Read the model definition and answer for the solid it produces. Units are mm, in the model's axes. Face numbers are marked on the shaded views. A direction names the side the tool comes from. Coordinates: 2 decimals unless noted, no trailing zeros. Loops run counter-clockwise (first coordinate to the right, second up) from the corner with the lowest first, then second, coordinate; pieces in that order, holes last.
from build123d import *

# Parameters (mm, degrees)
F0_W     = 127
F0_H     = 38.1
F1_DEPTH = 25.4
F4_DEPTH = 38.1
F5_DEPTH = 38.1
F3_R     = 6.35
F6_DEPTH = 25.4


with BuildPart() as f1:
    # F0 (on Top) → F1 (new body)
    with BuildSketch(Plane.XY):
        with Locations((3.767781, -13.309208)):
            Rectangle(F0_W, F0_H)
    extrude(amount=F1_DEPTH)

    # F2 (on face) → F4 (join)
    with BuildSketch(Plane.XZ.offset(32.359208)):
        with BuildLine():
            Line((-25.331575, 25.4), (-8.932219, 25.4))
            ThreePointArc((-8.932219, 25.4), (3.767781, 38.1), (16.467781, 25.4))
            Line((16.467781, 25.4), (32.867137, 25.4))
            ThreePointArc((32.867137, 25.4), (25.91106, 27.474418), (21.227394, 33.02))
            ThreePointArc((21.227394, 33.02), (3.767781, 44.45), (-13.691832, 33.02))
            ThreePointArc((-13.691832, 33.02), (-18.375498, 27.474418), (-25.331575, 25.4))
        make_face()
    extrude(amount=-F4_DEPTH)

    # F2 (on face) → F5 (cut)
    with BuildSketch(Plane.XZ.offset(32.359208)):
        with BuildLine():
            ThreePointArc((-8.932219, 25.4), (-5.212475, 16.419744), (3.767781, 12.7))
            Line((3.767781, 12.7), (3.767781, 25.4))
            Line((3.767781, 25.4), (-8.932219, 25.4))
        make_face()
        with BuildLine():
            Line((3.767781, 25.4), (3.767781, 12.7))
            ThreePointArc((3.767781, 12.7), (12.748037, 16.419744), (16.467781, 25.4))
            Line((16.467781, 25.4), (3.767781, 25.4))
        make_face()
    extrude(amount=-F5_DEPTH, mode=Mode.SUBTRACT)

    # F3 (on face) → F6 (cut)
    with BuildSketch(Plane.XY.offset(25.4)):
        with Locations((-40.682219, -13.309208)):
            Circle(F3_R)
        with Locations((48.217781, -13.309208)):
            Circle(F3_R)
    extrude(amount=-F6_DEPTH, mode=Mode.SUBTRACT)


solid = f1.part
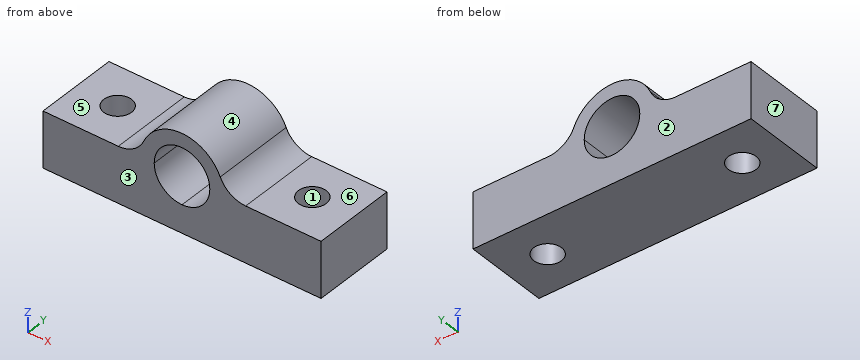
Q1. A cutting plane is placed at C-C (x = -4.5). Give the vertices of the cut face in (y, z).
Findings below:
outline: (-32.36, 0) - (5.74, 0) - (5.74, 15.76) - (-32.36, 15.76) - close; (-32.36, 35.04) - (5.74, 35.04) - (5.74, 42.56) - (-32.36, 42.56) - close
Q2. A cutting plane is placed at D-D (y = -28). Give the vertices of the cut face in (x, z).
Findings below:
outline: (-59.73, 0) - (67.27, 0) - (67.27, 25.4) - (32.87, 25.4) arc R12.7 cw to (21.23, 33.02) arc R19.05 ccw to (-13.69, 33.02) arc R12.7 cw to (-25.33, 25.4) - (-59.73, 25.4) - close; hole circle Ø25.4 at (3.77, 25.4)
Q3. A cutting plane is placed at B-B (z = 30.5). Give the vertices of the cut face in (x, y).
Findings below:
outline: (-15.16, -32.36) - (-7.86, -32.36) - (-7.86, 5.74) - (-15.16, 5.74) - close; (15.4, -32.36) - (22.69, -32.36) - (22.69, 5.74) - (15.4, 5.74) - close
Q4. Determine the mould class of the marked faces 1, 2, 3 and 4 for opening direction Y: +Y half, -Y half, draft (parallel to the pull), parting line (faces both ways), or undercut.
Findings below:
face 1: undercut
face 2: +Y half
face 3: -Y half
face 4: draft
Q5. Which of the six approach directions +Z, -Z, +X, -X, +Y, -Y give full straight-line access (tool end or side, diameter ignored) to the marked faces 5, 6 and 7?
Findings below:
face 5: +Z, -X, +Y, -Y
face 6: +Z, +X, +Y, -Y
face 7: +Z, -Z, -X, +Y, -Y
Q6. Flat-ended cylindrical pins translate along their axes: pin 1 Ø4 at (y, z) = (-22.5, 39) entering from -X; pin 2 Ø10 at (x, y) = (-37.5, 0.5) entering from +Z; pin 3 Ø7.5 at (x, y) = (48.22, -13.31) entering from +Z; pin 4 Ø6 at (y, z) = (-19, 32.5) entering from -X. Find the tip coordinate at first contact, or state that the pin passes through.
Findings below:
pin 1: stops at x = -11.34
pin 2: stops at z = 25.4
pin 3: passes through
pin 4: stops at x = -15.99
Q7. A cutting plane is placed at A-A (y = -8.5). Give the vertices of the cut face in (x, z).
Findings below:
outline: (-59.73, 0) - (-44.83, 0) - (-44.83, 25.4) - (-59.73, 25.4) - close; (-36.54, 0) - (44.07, 0) - (44.07, 25.4) - (32.87, 25.4) arc R12.7 cw to (21.23, 33.02) arc R19.05 ccw to (-13.69, 33.02) arc R12.7 cw to (-25.33, 25.4) - (-36.54, 25.4) - close; (52.36, 0) - (67.27, 0) - (67.27, 25.4) - (52.36, 25.4) - close; hole circle Ø25.4 at (3.77, 25.4)
Q8. Straight lines are drawn through the part: probe 1 along X at (y, z) = (-7.5, 12); probe 2 along Z at (x, y) = (42, -2); probe 3 along X at (y, z) = (1, 15.5). For each, find the intervals that lie inside material, in ascending order.
Findings below:
probe 1: x = -59.73 to -43.25, -38.12 to 45.65, 50.78 to 67.27
probe 2: z = 0 to 25.4
probe 3: x = -59.73 to -4.19, 11.72 to 67.27
